Check sheet for the drawn part. Datum: minimum x, y, z corner. Units: mm. Round coordinates to 2 decimals unless told otherwise and drop trailing zeros. Write each loop counter-clockwise with the first axis right and the second up, starting at its lowest first coordinate (ties: lowest second). Pieces come first, ordered by that corner, then holes. Notation, with made-up numbers: (19.5, 64) - (66.5, 64) arc R31 ccw to (66.5, 101) - close; hole circle Ø1 at (33, -23.75). An arc over 180 degrees is marked (long way). Answer as a JSON object with one key per item and string values. Group by question number.
1) Section check A-A (x = 235). Enter the section's corners in (y, z).
2) Section check C-C (y = 0.6). Enter the section's corners in (x, z), then the cut area to 3 significant figures.
3) Thickness scan on line 1 (Z direction, x = 175, y = 2.05); line 2 (X direction, y = 0.85, z = 175); line 3 (X direction, y = 2.35, z = 148). Record the ranges inside material, lowest first.
4) Go/stop test with a flat-tipped pin: pin 1 Ø1.5 at (y, z) = (2, 189) entering from -X. Record where the tip stops, or that it passes through.
5) Section check B-B (z = 310.5). Enter the section's corners in (x, y).
6) Section check D-D (z = 175). Enter the section's corners in (x, y), then the cut area to 3 significant figures.
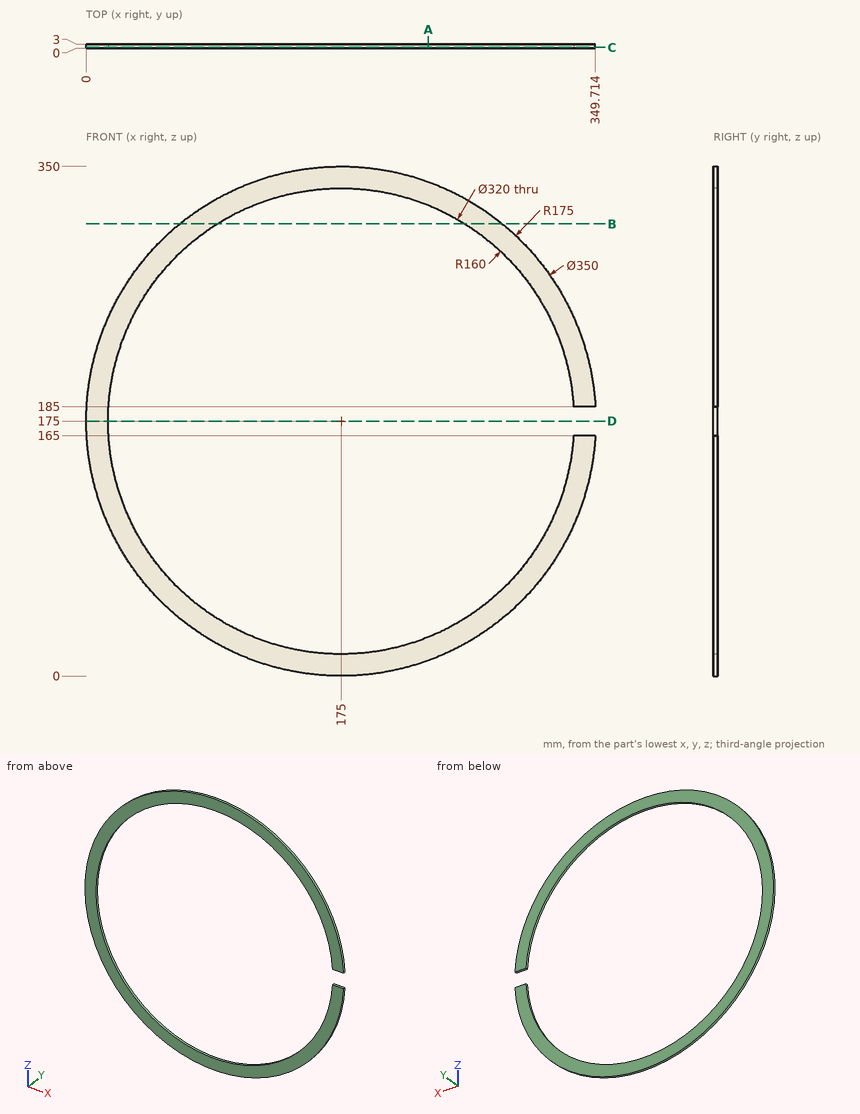
Returned:
{
 "1": {"outline": "(0, 10.61) - (3, 10.61) - (3, 26.68) - (0, 26.68) - close; (0, 323.32) - (3, 323.32) - (3, 339.39) - (0, 339.39) - close"},
 "2": {"outline": "(334.69, 165) arc R160 cw (long way) to (334.69, 185) - (349.71, 185) arc R175 ccw (long way) to (349.71, 165) - close", "area": "15,500 mm2"},
 "3": {"line 1": "0 to 15, 335 to 350", "line 2": "0 to 15", "line 3": "2.1 to 17.29, 332.71 to 347.9"},
 "4": {"pin 1": "x = 0.5"},
 "5": {"outline": "(64.25, 0) - (89.91, 0) - (89.91, 3) - (64.25, 3) - close; (260.09, 0) - (285.75, 0) - (285.75, 3) - (260.09, 3) - close"},
 "6": {"outline": "(0, 0) - (15, 0) - (15, 3) - (0, 3) - close", "area": "45.0 mm2"}
}
